The listing builds one solid part. Answer for the finished solid, in the listing's coordinates (mm). A direction names the side the tool comes from. Round coordinates to 2 decimals unless told otherwise and drop trailing zeros. Order: outer loops, then holes, each group sorted by start corner. A loop starts at its lowest first (then second) coordinate and runs counter-clockwise, first axis right, second up. Notation, with made-up numbers: M 36,-21 L 50,-21 A24 cw 50,1 Z; hole C -11.75,77.25 d5. An arc over 180 degrees is marked long. Put each result on its own line as item: value. Start each with the question number.
1. The part is cut by section A-A (z = 3.1). Count the separate pieces of the cut face and the enclosed holes in it, then the cut area to 3 significant figures.
2. The part is cut by section B-B (x = 0.75). Give the vertices of the cut face in (y, z).
3. Consider line 1 (Y direction, x = -0.75, z = 3.5); line 2 (X direction, y = -3.25, z = 3.7); line 3 (Z direction, x = 0, y = -1). Determine where each line is inside the solid, lowest interval first.
4. The part is cut by section C-C (y = -4). Give the vertices of the cut face in (x, z), then the cut area to 3 significant figures.
5. The mould has two halves that part along X. Classify faces 1 (the face through (-3.65, 0.66, 2.99)), 2 (the face through (-2.5, -5.5, 3)), 3 (the face through (-2.5, 5.5, 3)), 4 (the face through (0, 6, 4)): +X half, -X half, draft (parallel to the pull), parting line (faces both ways), or undercut.
6. Each of these flat-tipped pins is pushed along its axis until it touches: pin 1 Ø1.6 at (y, z) = (-2, 3) entering from +X; pin 2 Ø0.6 at (y, z) = (-3, 2.5) entering from -X; pin 3 Ø0.6 at (x, z) = (-0.5, 2.5) entering from +Y. Where does it stop, or does it pass through?
7. The part is cut by section D-D (y = 4.25). Give the vertices of the cut face in (x, z).
8. Which of the six approach directions +Z, -Z, +X, -X, +Y, -Y give full straight-line access (tool end or side, diameter ignored) to faces 5 (the face through (-2.634, 5.352, 2.986)), 6 (the face through (4, -5, 3)), 7 (the face through (0, 7, 3)), 8 (the face through (2.5, 5.5, 3)), 9 (the face through (-2.5, 6.5, 3))?
from build123d import *

# Parameters (mm, degrees)
F0_W     = 10
F0_H     = 16
F1_DEPTH = 2
F3_DEPTH = 2


# Not quite as in the source:
# - ends of sketch curves that miss each other by under 0.0002 mm in the source are joined
# - a feature names something its author has since deleted; it is built from what else it names


with BuildPart() as f1:
    # F0 (on Top) → F1 (new body)
    with BuildSketch(Plane.XY):
        Rectangle(F0_W, F0_H)
    extrude(amount=F1_DEPTH)

    # F2 (on face) → F3 (join)
    with BuildSketch(Plane.XY.offset(2)):
        Polygon((0, 7), (-2, 7), (-3, 6), (-2, 5), (0, 5), (2, 5), (3, 6), (2, 7), align=None)
        Polygon((-2.1414213562, 4.8585786438), (-3.1414213562, 5.8585786438), (-4.1414213562, 4.8585786438), (-4.1414213562, 1.1507223826), (-3.1374518146, 0.1453992321), (-2.1414213562, 1.0335195075), align=None)
        Polygon((2, 0.891659756), (2.00782e-05, 0.9006214721), (-2, 0.891659756), (-3, 0), (-2, -0.891659756), (-2.00782e-05, -0.9006214721), (2, -0.891659756), (3, 0), align=None)
        Polygon((3.1374518146, -0.1453992321), (2.1414213562, -1.0335195075), (2.1414213562, -4.8585786438), (3.1414213562, -5.8585786438), (4.1414213562, -4.8585786438), (4.1414213562, -1.1507223826), align=None)
        Polygon((0, -5), (-2, -5), (-3, -6), (-2, -7), (0, -7), (2, -7), (3, -6), (2, -5), align=None)
        Polygon((-4.1414213562, -4.8585786438), (-3.1414213562, -5.8585786438), (-2.1414213562, -4.8585786438), (-2.1414213562, -1.0335195075), (-3.1374518146, -0.1453992321), (-4.1414213562, -1.1507223826), align=None)
    extrude(amount=F3_DEPTH)


solid = f1.part
Resolved:
1. separate pieces: 6
1. enclosed holes: 0
1. area: 57.4 mm2
2. outline: M -8,0 L 8,0 L 8,2 L 7,2 L 7,4 L 5,4 L 5,2 L 0.9,2 L 0.9,4 L -0.9,4 L -0.9,2 L -5,2 L -5,4 L -7,4 L -7,2 L -8,2 Z
3. line 1: -7 to -5, -0.9 to 0.9, 5 to 7
3. line 2: -4.14 to -2.14, 2.14 to 4.14
3. line 3: 0 to 2
4. outline: M -5,0 L 5,0 L 5,2 L 4.14,2 L 4.14,4 L 2.14,4 L 2.14,2 L -2.14,2 L -2.14,4 L -4.14,4 L -4.14,2 L -5,2 Z
4. area: 28.0 mm2
5. face 1: -X half
5. face 2: undercut
5. face 3: undercut
5. face 4: draft
6. pin 1: x = 4.14
6. pin 2: x = -4.14
6. pin 3: y = 7
7. outline: M -5,0 L 5,0 L 5,2 L -2.14,2 L -2.14,4 L -4.14,4 L -4.14,2 L -5,2 Z
8. face 5: +Z
8. face 6: +Z, +X, -Y
8. face 7: +Z, +X, -X, +Y
8. face 8: +Z, +X
8. face 9: +Z, -X, +Y
